The listing builds one solid part. Answer for the finished solid, in the listing's coordinates (mm). A direction names the side the tool comes from. Coordinates: 2 decimals unless noted, no trailing zeros. Order: outer loops, then holes, each group sorted by start corner. A loop starts at its lowest first (then second) coordinate and runs counter-clockwise, first axis right, second up.
```python
from build123d import *

# Parameters (mm, degrees)
F1_DEPTH = 7.67
F2_DEPTH = 3.63
F4_DEPTH = 4.25
F5_DEPTH = 4.15


with BuildPart() as f1:
    # F0 (on Top) → F1 (new body)
    with BuildSketch(Plane.XY):
        with BuildLine():
            ThreePointArc((1.8, 19.6125731356), (-14.5489522819, -13.27482627), (19.695, 0))
            ThreePointArc((19.695, 0), (15.3557281657, 12.3326654662), (4.25, 19.2309782642))
            ThreePointArc((4.25, 19.2309782642), (3.0310111616, 19.4603698921), (1.8, 19.6125731356))
        make_face()
    extrude(amount=F1_DEPTH)

    # F0 (on Top) → F2 (join)
    with BuildSketch(Plane.XY):
        with BuildLine():
            ThreePointArc((1.8, 19.6125731356), (3.0310111616, 19.4603698921), (4.25, 19.2309782642))
            Line((4.25, 19.2309782642), (4.25, 24.6809782642))
            Line((4.25, 24.6809782642), (-4.03, 24.6809782642))
            Line((-4.03, 24.6809782642), (-4.03, 20.3809782642))
            Line((-4.03, 20.3809782642), (-1.58, 20.3809782642))
            Line((-1.58, 20.3809782642), (-1.58, 22.2309782642))
            Line((-1.58, 22.2309782642), (1.8, 22.2309782642))
            Line((1.8, 22.2309782642), (1.8, 19.6125731356))
        make_face()
    extrude(amount=F2_DEPTH)

    # F3 (on face) → F4 (cut)
    with BuildSketch(Plane.XY.offset(7.67)):
        Polygon((4.2250477709, 3.83), (4.2250477709, 6.68), (-4.2250477709, 6.68), (-4.2250477709, 3.83), (-4.2250477709, -3.83), (-4.2250477709, -6.68), (4.2250477709, -6.68), (4.2250477709, -3.83), align=None)
    extrude(amount=-F4_DEPTH, mode=Mode.SUBTRACT)

    # F3 (on face) → F5 (cut)
    with BuildSketch(Plane.XY.offset(7.67)):
        with BuildLine():
            Line((-4.2250477709, -3.83), (-4.2250477709, 3.83))
            Line((-4.2250477709, 3.83), (-19.3190094208, 3.83))
            ThreePointArc((-19.3190094208, 3.83), (-19.695, 0), (-19.3190094208, -3.83))
            Line((-19.3190094208, -3.83), (-4.2250477709, -3.83))
        make_face()
        with BuildLine():
            Line((19.3190094208, 3.83), (4.2250477709, 3.83))
            Line((4.2250477709, 3.83), (4.2250477709, -3.83))
            Line((4.2250477709, -3.83), (19.3190094208, -3.83))
            ThreePointArc((19.3190094208, -3.83), (19.6007769686, -1.9242056098), (19.695, 0))
            ThreePointArc((19.695, 0), (19.6007769686, 1.9242056098), (19.3190094208, 3.83))
        make_face()
    extrude(amount=-F5_DEPTH, mode=Mode.SUBTRACT)


solid = f1.part
```
1) For faces 1 (the flat face through (12, 3.83, 6)), 2 (the flat face through (0, -6.68, 6)), 3 (the flat face through (4.25, 22, 2)), 4 (the flat face through (-1.58, 21, 2)), determine the directions among +Z, -Z, +X, -X, +Y, -Y from which every point of the face is accessible in a straight line to the end or side of a thin tool.
2) A cutting plane is placed at D-D, the plane z = 2.5. Write down the section's boundary in (x, y) (3 decimals).
3) Each of these flat-tipped pins is pushed along its axis until it touches: P1, Ø2.5, axis at x = 1, z = 2.5, coming from the -Y side (3 decimals); P2, Ø3, axis at y = 23.5, z = 1, coming from the -X side; P3, Ø2, axis at x = -13.5, z = 5, coming from the -Y side; P4, Ø6, axis at x = 2, y = 23, coming from the +Z side. Where does it stop, or does it pass through?
4) Straight lines are drawn through the part: probe 1 along Z at (x, y) = (7.5, 2); probe 2 along Z at (x, y) = (0, 5); probe 3 along X at (y, z) = (-4.5, 5.75). For each, find the intervals that lie inside material, in ascending order.
5) A cutting plane is placed at A-A, the plane x = 0. Write down the section's boundary in (y, z) (3 decimals), plus the area to 3 significant figures.
6) A cutting plane is placed at C-C, the plane y = 3. Write down the section's boundary in (x, z).
7) A cutting plane is placed at B-B, the plane z = 5.5. Write down the section's boundary in (x, y) (3 decimals).
Working result:
1. face 1: +Z, +X, -X
1. face 2: +Z
1. face 3: +Z, -Z, +X, +Y
1. face 4: +Z, -Z
2. outline: (-4.03, 20.381) - (-1.58, 20.381) - (-1.58, 22.231) - (1.8, 22.231) - (1.8, 19.613) arc R19.695 ccw (long way) to (4.25, 19.231) - (4.25, 24.681) - (-4.03, 24.681) - close
3. P1: stops at y = -19.695
3. P2: stops at x = -4.03
3. P3: stops at y = -15.22
3. P4: stops at z = 3.63
4. probe 1: z = 0 to 3.52
4. probe 2: z = 0 to 3.42
4. probe 3: x = -19.17 to -4.23, 4.23 to 19.17
5. outline: (-19.695, 0) - (19.695, 0) - (19.695, 7.67) - (6.68, 7.67) - (6.68, 3.42) - (-6.68, 3.42) - (-6.68, 7.67) - (-19.695, 7.67) - close; (22.231, 0) - (24.681, 0) - (24.681, 3.63) - (22.231, 3.63) - close
5. area: 254 mm2
6. outline: (-19.47, 0) - (19.47, 0) - (19.47, 3.52) - (4.23, 3.52) - (4.23, 3.42) - (-4.23, 3.42) - (-4.23, 3.52) - (-19.47, 3.52) - close
7. outline: (-19.319, -3.83) arc R19.695 ccw to (19.319, -3.83) - (4.225, -3.83) - (4.225, -6.68) - (-4.225, -6.68) - (-4.225, -3.83) - close; (-19.319, 3.83) - (-4.225, 3.83) - (-4.225, 6.68) - (4.225, 6.68) - (4.225, 3.83) - (19.319, 3.83) arc R19.695 ccw to start
